Design review of the part built by this model. Coordinates are the model's own, in mm. A direction names the side the tool comes from. Coordinates: 2 decimals unless noted, no trailing zeros. Write each loop counter-clockwise with the first axis right and the second up, starting at its lowest first coordinate (ties: lowest second). Pieces come first, ordered by that corner, then holes.
Q1. Take a section at C-C, the plane x = 190. Write out the cut boundary in (y, z).
Q2. For L1, parallel to X at y = 52, z = 7.5; L2, parallel to Y at x = 70, z = 19.5; L3, parallel to Y at x = 178, z = 25.5, list the stretches that pass through material, from the lowest coordinate up.
Q3. For faces 4 (the flat face through (101, 137, 20)), 5 (the flat face through (84, 88.25, 21)), list the 3-axis set-ups (+Z, -Z, +X, -X, +Y, -Y) from which the entire face can be reached by the end or side of a thin tool; tool diameter is ignored.
Q4. The part is to be moulded in two halves that separate along X. For faces 1 (the flat face through (29, 110, 41)), 2 (the flat face through (2, 110, 21)), 3 (the flat face through (210, 65, 20)), say which applies: released by +X, released by -X, zero draft, split by the parting line, or undercut.
Q5. Take a section at B-B, the plane y = 92.5. Write out the cut boundary in (x, z).
Q6. Take a section at A-A, the plane z = 17.5. State how many separate pieces and enclosed holes the cut face has, plus the area to 3 significant figures.
from build123d import *

# Parameters (mm, degrees)
ESQUISSE1_W                     = 205
ESQUISSE1_H                     = 132
BOSS_EXTRU_1_DEPTH              = 1
ESQUISSE1_2_W                   = 215
ESQUISSE1_2_H                   = 142
ESQUISSE1_2_W_2                 = 205
ESQUISSE1_2_H_2                 = 132
EXTRU_MINCE1_DEPTH              = 40
ESQUISSE2_W                     = 54
ESQUISSE2_H                     = 43.5
BOSS_EXTRU_2_DEPTH              = 40
R_P_TITION_LIN_AIRE1_COUNT      = 3
R_P_TITION_LIN_AIRE1_PITCH      = 43.75
R_P_TITION_LIN_AIRE1_COUNT_DIR2 = 2
R_P_TITION_LIN_AIRE1_PITCH_DIR2 = 55


with BuildPart() as part:
    # Esquisse1 → Boss.-Extru.1 (new body)
    with BuildSketch(Plane.XY):
        with Locations((102.5, 66)):
            Rectangle(ESQUISSE1_W, ESQUISSE1_H)
    extrude(amount=BOSS_EXTRU_1_DEPTH)

    # Esquisse1<2> → Extru.-Mince1 (add)
    with BuildSketch(Plane.XY):
        with Locations((102.5, 66)):
            Rectangle(ESQUISSE1_2_W, ESQUISSE1_2_H)
        with Locations((102.5, 66)):
            Rectangle(ESQUISSE1_2_W_2, ESQUISSE1_2_H_2, mode=Mode.SUBTRACT)
    extrude(amount=EXTRU_MINCE1_DEPTH)

    # Esquisse2 → Boss.-Extru.2 (add)
    with BuildSketch(Plane.XY.offset(1)):
        with Locations((29, 110)):
            Rectangle(ESQUISSE2_W, ESQUISSE2_H)
    boss_extru_2 = extrude(amount=BOSS_EXTRU_2_DEPTH)

    # Répétition linéaire1: Boss.-Extru.2 3 × 2
    with Locations(*[(j * R_P_TITION_LIN_AIRE1_PITCH_DIR2, -i * R_P_TITION_LIN_AIRE1_PITCH, 0) for i in range(R_P_TITION_LIN_AIRE1_COUNT) for j in range(R_P_TITION_LIN_AIRE1_COUNT_DIR2) if (i, j) != (0, 0)]):
        add(boss_extru_2)


solid = part.part
Responses:
1. outline: (-5, 0) - (137, 0) - (137, 40) - (132, 40) - (132, 1) - (0, 1) - (0, 40) - (-5, 40) - close
2. L1: x = -5 to 0, 2 to 56, 57 to 111, 205 to 210
2. L2: y = -5 to 0, 0.75 to 44.25, 44.5 to 88, 88.25 to 131.75, 132 to 137
2. L3: y = -5 to 0, 132 to 137
3. face 4: +Z, -Z, +X, -X, +Y
3. face 5: +Z
4. face 1: zero draft
4. face 2: undercut
4. face 3: released by +X
5. outline: (-5, 0) - (210, 0) - (210, 40) - (205, 40) - (205, 1) - (111, 1) - (111, 41) - (57, 41) - (57, 1) - (56, 1) - (56, 41) - (2, 41) - (2, 1) - (0, 1) - (0, 40) - (-5, 40) - close
6. separate pieces: 7
6. enclosed holes: 1
6. area: 17,600 mm2
